Build history of the part. All positions in model axes, mm. Face numbers are marked on the shaded views. A direction names the side the tool comes from. Round coordinates to 2 decimals unless told otherwise and drop trailing zeros. Order: outer loops, then holes, each group sorted by start corner. A loop starts at its lowest first (then second) coordinate and runs counter-clockwise, first axis right, second up. Notation, with made-up numbers: (-29.5, 66.25) -> (-1.5, 66.25) arc R23 cw to (-1.5, 87.25) -> close; hole circle Ø1 at (-21.5, 16). An arc over 180 degrees is marked (long way). Answer as a JSON object with one key per item and string values.
from build123d import *

# Parameters (mm, degrees)
SALIENTE_EXTRUIR1_DEPTH = 175
REDONDEO1_R             = 5


with BuildPart() as part:
    # Croquis1 → Saliente-Extruir1 (new, symmetric)
    with BuildSketch(Plane(origin=(0, 0, 0), x_dir=(0, 0, -1), z_dir=(1, 0, 0))):
        Polygon((74.427480916, 0), (-74.427480916, 0), (-74.427480916, 20), (-15, 20), (-15, 30), (15, 30), (15, 20), (74.427480916, 20), align=None)
    extrude(amount=SALIENTE_EXTRUIR1_DEPTH, both=True)

    # Redondeo1
    redondeo1_edges = [part.edges().sort_by_distance(p)[0] for p in [
        (-175, 25, -15),
        (-175, 20, -44.713740458),
        (175, 25, -15),
        (0, 20, 74.427480916),
        (0, 20, 15),
        (0, 20, -15),
        (0, 20, -74.427480916),
        (175, 25, 15),
        (175, 20, 44.713740458),
        (175, 20, -44.713740458),
        (-175, 20, 44.713740458),
        (-175, 25, 15),
    ]]
    fillet(redondeo1_edges, radius=REDONDEO1_R)


solid = part.part
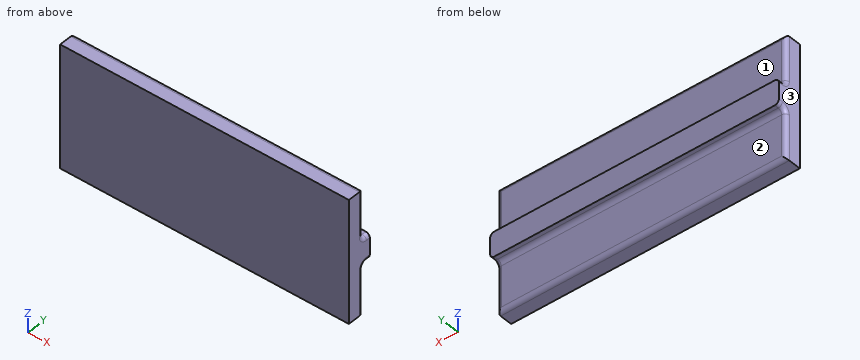
1) Probe L1, parallel to Y at x = -8.5, z = -37; L2, parallel to Z at x = -55.5, y = 26.5; L3, parallel to Z at x = -21.5, y = 15.5. List the from-to ranges inside material, lowest first. Write a range as from..to.
Checked values:
{"L1": "y = 0..20", "L2": "z = -15..15", "L3": "z = -74.4..74.4"}
2) Cut at A-A, the plane x = -6. Give the cut face in (y, z), plus the area to 3 significant figures.
Checked values:
{"outline": "(0, -74.43) -> (15, -74.43) arc R5 ccw to (20, -69.43) -> (20, -20) arc R5 cw to (25, -15) -> (30, -15) -> (30, 15) -> (25, 15) arc R5 cw to (20, 20) -> (20, 69.43) arc R5 ccw to (15, 74.43) -> (0, 74.43) -> close", "area": "3,280 mm²"}
3) Cut at B-B, the plane z = -54. Give the cut face in (x, y), plus the area to 3 significant figures.
Checked values:
{"outline": "(-175, 0) -> (175, 0) -> (175, 15) arc R5 ccw to (170, 20) -> (-170, 20) arc R5 ccw to (-175, 15) -> close", "area": "6,990 mm²"}
4) Which spindle directions (+Z, -Z, +X, -X, +Y, -Y) get a long thin tool onto all of the face, cutting with end or side? Do the marked faces 1, 2 and 3. Say none if no direction does.
Checked values:
{"face 1": "+Z, +X, -X, +Y", "face 2": "-Z, +X, -X, +Y", "face 3": "+Z, -Z, -X, +Y, -Y"}
5) Flat gauge pins, fed straight in: pin 1 Ø8 at (x, y) = (-99.5, 19.5) entering from -Z; pin 2 Ø5.5 at (x, y) = (-19, 27.5) entering from +Z; pin 3 Ø5 at (y, z) = (19, 53.5) entering from +X. Where does each tip first touch, or does it go through?
Checked values:
{"pin 1": "stops at z = -74.4", "pin 2": "stops at z = 15.01", "pin 3": "stops at x = 174.77"}
